Geometry: see drawing. Coordinates: mm, zero at the bounding-box minimum. A direction names the side the tool comes from. Coordinates: 2 decimals unless noted, no trailing zeros. Order: outer loops, then holes, each group sorted by start corner. A loop starts at its lowest first (then second) coordinate and runs counter-clockwise, first axis right, second up. Notation, with made-up numbers: (85.25, 70.25) - (121.25, 70.25) arc R18 ccw to (121.25, 98.25) - close; hole circle Ø8 at (70, 27.5). An arc over 180 degrees is marked (long way). Use a Markdown table: item, result. Add a question column.
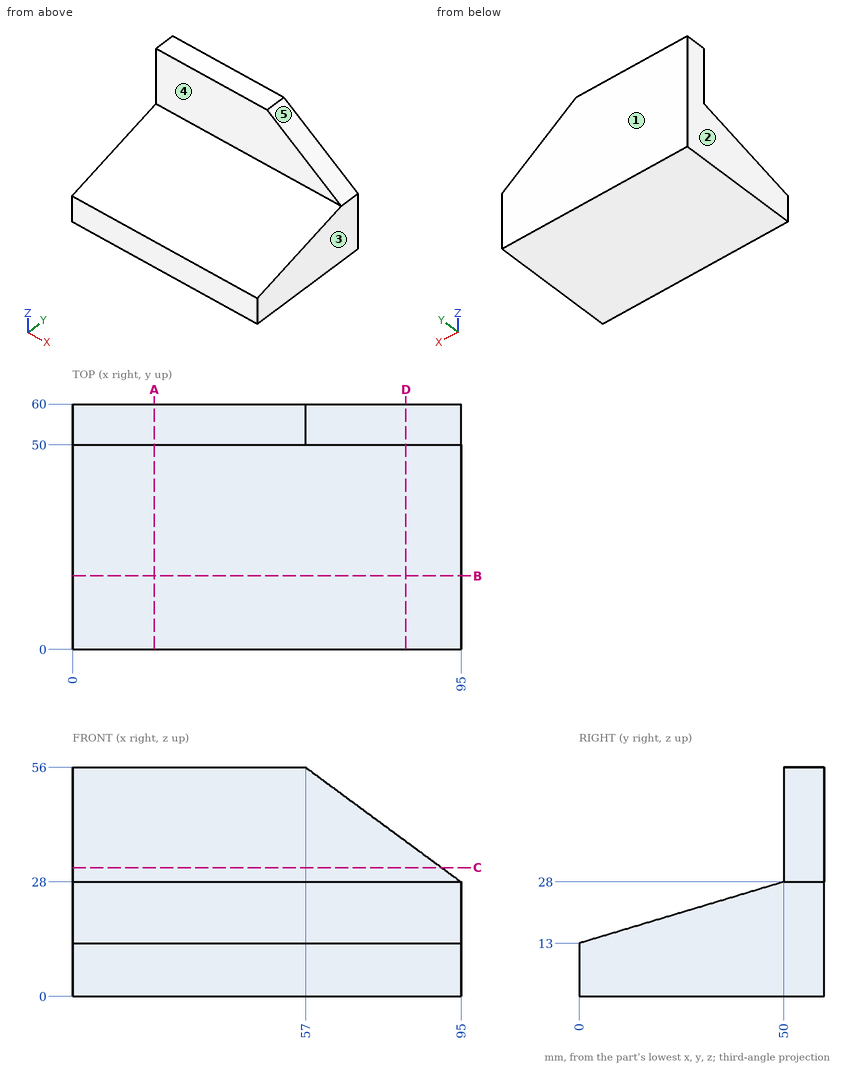
1) Section query C-C (z = 31.5). Return the cut outline in (x, y), and give its area (4 significant figures).
2) Draft query along X for the marked faces 1, 2 and 3. Return one class per face: released by +X, released by -X, zero draft, split by the parting line, or undercut.
3) Section query D-D (x = 81.5). Return the cut outline in (y, z).
4) First-contact query: pin 1 (8 mm diameter, centred on y = 50, z = 40, fed in from +X); pin 2 (4 mm diameter, centred on x = 50.5, z = 48.5, fed in from -Y); pin 3 (5 mm diameter, centred on x = 19.5, y = 33, fed in from -Z); pin 4 (1.5 mm diameter, centred on x = 45, y = 44, fed in from +Z) (3 decimals). Flat tips, straight axial feed; report the tip coordinate or a pass-through.
5) Access query for the marked faces 4 and 5. Directions: +Z, -Z, +X, -X, +Y, -Y. A direction counts if a zero-diameter tool reaches every point of the face in a straight line with its end or side. Return the directions, or none.
6) Line query: line 1 (Y direction, x = 55.5, z = 35); line 2 (Z direction, x = 75, y = 24.5); line 3 (Z direction, x = 91.5, y = 49). Output: solid intervals per line, ascending. Write a range as from..to.
7) Section query B-B (y = 18). Return the cut outline in (x, z).
8) Section query A-A (x = 20). Return the cut outline in (y, z), and give its area (4 significant figures).
From the geometry:
| question | item | result |
|---|---|---|
| 1 | outline | (0, 50) - (90.25, 50) - (90.25, 60) - (0, 60) - close |
| 1 | area | 902.5 mm^2 |
| 2 | face 1 | zero draft |
| 2 | face 2 | released by -X |
| 2 | face 3 | released by +X |
| 3 | outline | (0, 0) - (60, 0) - (60, 37.95) - (50, 37.95) - (50, 28) - (0, 13) - close |
| 4 | pin 1 | stops at x = 84.14 |
| 4 | pin 2 | stops at y = 50 |
| 4 | pin 3 | stops at z = 0 |
| 4 | pin 4 | stops at z = 26.425 |
| 5 | face 4 | +Z, +X, -X, -Y |
| 5 | face 5 | +Z, +X, +Y, -Y |
| 6 | line 1 | y = 50..60 |
| 6 | line 2 | z = 0..20.35 |
| 6 | line 3 | z = 0..27.7 |
| 7 | outline | (0, 0) - (95, 0) - (95, 18.4) - (0, 18.4) - close |
| 8 | outline | (0, 0) - (60, 0) - (60, 56) - (50, 56) - (50, 28) - (0, 13) - close |
| 8 | area | 1,585 mm^2 |
